```python
from build123d import *

# Parameters (mm, degrees)
EXTRUDE_START      = 345
EXTRUDE_SKETCH_1_W = 160
EXTRUDE_SKETCH_1_H = 100
EXTRUDE_1_DEPTH    = 1.6
EXTRUDE_START_2    = 346.6
EXTRUDE_SKETCH_2_W = 25
EXTRUDE_SKETCH_2_H = 18
EXTRUDE_2_DEPTH    = 3
EXTRUDE_SKETCH_3_W = 40
EXTRUDE_SKETCH_3_H = 40
EXTRUDE_3_DEPTH    = 4
EXTRUDE_SKETCH_4_W = 23
EXTRUDE_SKETCH_4_H = 20
EXTRUDE_4_DEPTH    = 2.4
EXTRUDE_START_3    = 323
EXTRUDE_SKETCH_5_R = 3
EXTRUDE_5_DEPTH    = 22
EXTRUDE_SKETCH_6_R = 3
EXTRUDE_6_DEPTH    = 22
EXTRUDE_SKETCH_7_R = 3
EXTRUDE_7_DEPTH    = 22
EXTRUDE_SKETCH_8_R = 3
EXTRUDE_8_DEPTH    = 22


with BuildPart() as part:
    # Extrude sketch 1 → Extrude 1 (new body)
    with BuildSketch(Plane.XY.offset(EXTRUDE_START)):
        with Locations((557, 55)):
            Rectangle(EXTRUDE_SKETCH_1_W, EXTRUDE_SKETCH_1_H)
    extrude(amount=EXTRUDE_1_DEPTH)


with BuildPart() as body_2:
    # Extrude sketch 2 → Extrude 2 (new body)
    with BuildSketch(Plane.XY.offset(EXTRUDE_START_2)):
        with Locations((509.5, 39)):
            Rectangle(EXTRUDE_SKETCH_2_W, EXTRUDE_SKETCH_2_H)
    extrude(amount=EXTRUDE_2_DEPTH)


with BuildPart() as body_3:
    # Extrude sketch 3 → Extrude 3 (new body)
    with BuildSketch(Plane.XY.offset(EXTRUDE_START_2)):
        with Locations((567, 65)):
            Rectangle(EXTRUDE_SKETCH_3_W, EXTRUDE_SKETCH_3_H)
    extrude(amount=EXTRUDE_3_DEPTH)


with BuildPart() as body_4:
    # Extrude sketch 4 → Extrude 4 (new body)
    with BuildSketch(Plane.XY.offset(EXTRUDE_START_2)):
        with Locations((613.5, 30)):
            Rectangle(EXTRUDE_SKETCH_4_W, EXTRUDE_SKETCH_4_H)
    extrude(amount=EXTRUDE_4_DEPTH)


with BuildPart() as body_5:
    # Extrude sketch 5 → Extrude 5 (new body)
    with BuildSketch(Plane.XY.offset(EXTRUDE_START_3)):
        with Locations((482, 10)):
            Circle(EXTRUDE_SKETCH_5_R)
    extrude(amount=EXTRUDE_5_DEPTH)


with BuildPart() as body_6:
    # Extrude sketch 6 → Extrude 6 (new body)
    with BuildSketch(Plane.XY.offset(EXTRUDE_START_3)):
        with Locations((482, 100)):
            Circle(EXTRUDE_SKETCH_6_R)
    extrude(amount=EXTRUDE_6_DEPTH)


with BuildPart() as body_7:
    # Extrude sketch 7 → Extrude 7 (new body)
    with BuildSketch(Plane.XY.offset(EXTRUDE_START_3)):
        with Locations((632, 10)):
            Circle(EXTRUDE_SKETCH_7_R)
    extrude(amount=EXTRUDE_7_DEPTH)


with BuildPart() as body_8:
    # Extrude sketch 8 → Extrude 8 (new body)
    with BuildSketch(Plane.XY.offset(EXTRUDE_START_3)):
        with Locations((632, 100)):
            Circle(EXTRUDE_SKETCH_8_R)
    extrude(amount=EXTRUDE_8_DEPTH)


with BuildPart() as body_5_1:
    add(body_5.part)

    # Combine (weld / assembly of features): union body 3, body 6, part, body 7, body 2, body 8, body 4
    add(body_3.part)
    add(body_6.part)
    add(part.part)
    add(body_7.part)
    add(body_2.part)
    add(body_8.part)
    add(body_4.part)


solid = body_5_1.part
```
For this review, take the finished solid that the model builds, in its own axes (mm). A direction names the side the tool comes from. Coordinates: 2 decimals unless noted, no trailing zeros. Write each loop counter-clockwise with the first axis right and the second up, starting at its lowest first coordinate (ties: lowest second). Pieces come first, ordered by that corner, then holes.
(1) Tool access review of faces 1 (the face through (587, 65, 349)), 2 (the face through (484.86, 10.9, 333.85)), 3 (the face through (509, 48, 348)): name each direction out of +Z, -Z, +X, -X, +Y, -Y from which nothing blocks a thin tool from reaching the whole face with its end or side.
(2) Add section B-B on y = 51.5. Give the boundary of the cut face in (x, z).
(3) Add section D-D on x = 632. Give the boundary of the cut face in (y, z).
(4) For pin 1 Ø0.9 at (y, z) = (42.5, 348.5) entering from -X; pin 2 Ø2.5 at (x, z) = (613.5, 348.5) entering from +Y; pin 3 Ø5.5 at (x, y) = (513.5, 38.5) entering from +Z, all flat-tipped, find the tip position at first contact; note any pin that passes through.
(5) Add section A-A on x = 520. Give the boundary of the cut face in (y, z).
(6) Wall thickness on probe 1 along X at (y, z) = (30.5, 348.5); probe 2 along Z at (x, y) = (536.5, 72.5); probe 3 along X at (y, z) = (9, 336.25): over which ranges is each line inside the solid? List them lowest first.
(7) The part is to be moulded in two halves that separate along X. For faces 4 (the face through (497, 39, 348)), 5 (the face through (522, 39, 348)), 6 (the face through (567, 45, 349)), say which applies: +X half, -X half, draft (parallel to the pull), parting line (faces both ways), or undercut.
(8) Add section C-C on z = 328.5. Give the boundary of the cut face in (x, y).
Answer sheet:
1. face 1: +Z, +X, +Y, -Y
1. face 2: -Z
1. face 3: +Z, -X, +Y
2. outline: (477, 345) - (637, 345) - (637, 346.6) - (587, 346.6) - (587, 350.6) - (547, 350.6) - (547, 346.6) - (477, 346.6) - close
3. outline: (5, 345) - (7, 345) - (7, 323) - (13, 323) - (13, 345) - (97, 345) - (97, 323) - (103, 323) - (103, 345) - (105, 345) - (105, 346.6) - (5, 346.6) - close
4. pin 1: stops at x = 497
4. pin 2: stops at y = 40
4. pin 3: stops at z = 349.6
5. outline: (5, 345) - (105, 345) - (105, 346.6) - (48, 346.6) - (48, 349.6) - (30, 349.6) - (30, 346.6) - (5, 346.6) - close
6. probe 1: x = 497 to 522, 602 to 625
6. probe 2: z = 345 to 346.6
6. probe 3: x = 479.17 to 484.83, 629.17 to 634.83
7. face 4: -X half
7. face 5: undercut
7. face 6: draft
8. outline: circle Ø6 at (482, 10); circle Ø6 at (482, 100); circle Ø6 at (632, 10); circle Ø6 at (632, 100)
